The model under review builds one solid part; all positions refer to its coordinate system, in mm. Face numbers are marked on the shaded views. A direction names the side the tool comes from. Round coordinates to 2 decimals unless told otherwise and drop trailing zeros. Write each loop counter-clockwise with the first axis right and the second up, starting at its lowest first coordinate (ties: lowest second). Pieces come first, ordered by that corner, then holes. Notation, with made-up numbers: (-19, -22) -> (-8, -22) arc R19 ccw to (-8, -1) -> close; hole circle Ø5 at (60.5, -38.5). An arc over 180 degrees is marked (long way). Return JSON: item names as keys, results as strings. Group by question number.
1. For line 1 along X through (y, z) = (2.25, -6.5); line 2 along X through (y, z) = (-6.5, 0); line 3 along Y through (x, z) = (-7, 4.5), list the stretches that pass through material, from the lowest coordinate up. Write a range as from..to.
2. Clearance check with flat-ended pins moving along their axes: P1, Ø1, axis at y = -4, z = 7, coming from the -X side; P2, Ø1.5, axis at x = 10, y = 3, coming from the +Z side; P3, Ø4, axis at x = 1.5, y = -2.5, coming from the -Z side; P4, Ø4.5, axis at x = 0, z = 0, coming from the +Y side. State where each tip first meets the part, or that it passes through.
3. Mouldability with a two-part tool opening along Z and no side actions: class the marked faces 1, 2 and 3 as pulls with the +Z half, pulls with the -Z half, needs draft (parallel to the pull), parting line crosses it, or undercut.
4. Take a section at A-A, the plane y = -2.25. Write out the cut boundary in (x, z).
5. Take a section at B-B, the plane z = -11.5. Write out the cut boundary in (x, y).
6. Tool access review of the marked faces 4, 5 and 6: name each direction out of +Z, -Z, +X, -X, +Y, -Y from which nothing blocks a thin tool from reaching the whole face with its end or side.
from build123d import *

# Parameters (mm, degrees)
SKETCH1_R                 = 17
BOSS_EXTRUDE1_DEPTH       = 14
SKETCH9_W                 = 6
SKETCH9_H                 = 13.19
CUT_EXTRUDE1_DEPTH        = 28.820855486
SKETCH10_R                = 2.5
CUT_EXTRUDE2_DEPTH        = 6.35
FILLET2_R                 = 1
CIRPATTERN2_COUNT         = 3
FILLET2_OF_CIRPATTERN2_R  = 1
SKETCH12_R                = 20
CUT_EXTRUDE3_DEPTH        = 10
BOSS_EXTRUDE2_START       = 1
SKETCH13_R                = 17
BOSS_EXTRUDE2_DEPTH       = 1
M2X0_4_TAPPED_HOLE3_D     = 1.6
M2X0_4_TAPPED_HOLE3_DEPTH = 7
M2X0_4_TAPPED_HOLE3_TIP   = 0.480688495
FILLET3_R                 = 1
SKETCH14_R                = 11
SKETCH14_R_2              = 9.652
BOSS_EXTRUDE3_DEPTH       = 7
SKETCH20_R                = 2.5
CUT_EXTRUDE5_DEPTH        = 8
FILLET4_R                 = 0.25


with BuildPart() as part:
    # Sketch1 → Boss-Extrude1 (new body)
    with BuildSketch(Plane(origin=(0, 0, 0), x_dir=(1, 0, 0), z_dir=(0, 1, 0))):
        with Locations(Location((0, 0, 0), (0, 0, 270))):
            Circle(SKETCH1_R)
    extrude(amount=BOSS_EXTRUDE1_DEPTH)

    # Sketch9 → Cut-Extrude1 (cut, through all)
    with BuildSketch(Plane(origin=(0, 14, 0), x_dir=(1, 0, 0), z_dir=(0, 1, 0))):
        with Locations((0, 10.405)):
            Rectangle(SKETCH9_W, SKETCH9_H)
    cut_extrude1 = extrude(amount=-CUT_EXTRUDE1_DEPTH, mode=Mode.SUBTRACT)

    # Sketch10 → Cut-Extrude2 (cut, symmetric)
    with BuildSketch(Plane(origin=(0, 0, 0), x_dir=(0, 0, -1), z_dir=(1, 0, 0))):
        with Locations((11.5, 7)):
            Circle(SKETCH10_R)
    cut_extrude2 = extrude(amount=CUT_EXTRUDE2_DEPTH, both=True, mode=Mode.SUBTRACT)

    # Fillet2
    fillet2_edges = [part.edges().sort_by_distance(p)[0] for p in [
        (-3, 7, -3.81),
        (3, 7, -3.81),
    ]]
    fillet(fillet2_edges, radius=FILLET2_R)

    # CirPattern2: Cut-Extrude1, Cut-Extrude2 ×3 about axis
    cirpattern2_axis = Axis((0, 0, 0), (0, 1, 0))
    add([cut_extrude1.rotate(cirpattern2_axis, i * 360 / CIRPATTERN2_COUNT) for i in range(1, CIRPATTERN2_COUNT)], mode=Mode.SUBTRACT)
    add([cut_extrude2.rotate(cirpattern2_axis, i * 360 / CIRPATTERN2_COUNT) for i in range(1, CIRPATTERN2_COUNT)], mode=Mode.SUBTRACT)

    # Fillet2 of CirPattern2
    fillet2_of_cirpattern2_edges = [part.edges().sort_by_distance(p)[0] for p in [
        (-1.799556788, 7, 4.503076211),
        (-4.799556788, 7, -0.693076211),
        (4.799556788, 7, -0.693076211),
        (1.799556788, 7, 4.503076211),
    ]]
    fillet(fillet2_of_cirpattern2_edges, radius=FILLET2_OF_CIRPATTERN2_R)

    # Sketch12 → Cut-Extrude3 (cut)
    with BuildSketch(Plane(origin=(0, 7, 0), x_dir=(1, 0, 0), z_dir=(0, 1, 0))):
        Circle(SKETCH12_R)
    extrude(amount=CUT_EXTRUDE3_DEPTH, mode=Mode.SUBTRACT)

    # Sketch13 → Boss-Extrude2 (add)
    with BuildSketch(Plane.XZ.offset(BOSS_EXTRUDE2_START)):
        with Locations(Location((0, 0, 0), (0, 0, 270))):
            Circle(SKETCH13_R)
    extrude(amount=-BOSS_EXTRUDE2_DEPTH)

    # M2x0.4 Tapped Hole3
    with Locations(Plane(origin=(0, 7, 0), x_dir=(1, 0, 0), z_dir=(0, 1, 0))):
        with Locations((-11.258330249, 6.5), (11.258330249, 6.5), (0, -13), (-7.361215932, 4.25), (7.361215932, 4.25), (0, -8.5)):
            Hole(M2X0_4_TAPPED_HOLE3_D / 2, depth=M2X0_4_TAPPED_HOLE3_DEPTH)
            with Locations((0, 0, -(M2X0_4_TAPPED_HOLE3_DEPTH + M2X0_4_TAPPED_HOLE3_TIP / 2))):  # 118° drill point
                Cone(0, M2X0_4_TAPPED_HOLE3_D / 2, M2X0_4_TAPPED_HOLE3_TIP, mode=Mode.SUBTRACT)

    # Fillet3
    fillet3_edges = [part.edges().sort_by_distance(p)[0] for p in [
        (-10.828479469, 0, 2.787723921),
        (-4.906763147, 0, -0.292976634),
        (-3.299556788, 0, 1.905),
        (-2.199656366, 0, 4.395869853),
        (7.828479469, 0, 7.983876344),
        (2.199656366, 0, 4.395869853),
        (10.828479469, 0, 2.787723921),
        (4.906763147, 0, -0.292976634),
        (-3, 0, -10.771600265),
        (-2.707106781, 0, -4.102893219),
        (0, 0, -3.81),
        (2.707106781, 0, -4.102893219),
        (-7.828479469, 0, 7.983876344),
        (3.299556788, 0, 1.905),
        (3, 0, -10.771600265),
    ]]
    fillet(fillet3_edges, radius=FILLET3_R)

    # Sketch14 → Boss-Extrude3 (add)
    with BuildSketch(Plane.XZ.offset(1)):
        with Locations(Location((0, 0, 0), (0, 0, 270))):
            Circle(SKETCH14_R)
        with Locations(Location((0, 0, 0), (0, 0, 270))):
            Circle(SKETCH14_R_2, mode=Mode.SUBTRACT)
    extrude(amount=BOSS_EXTRUDE3_DEPTH)

    # Sketch20 → Cut-Extrude5 (cut)
    with BuildSketch(Plane.XZ.offset(1)):
        with Locations(Location((0, 0, 0), (0, 0, 270))):
            Circle(SKETCH20_R)
    extrude(amount=-CUT_EXTRUDE5_DEPTH, mode=Mode.SUBTRACT)

    # Fillet4
    fillet4_edges = [part.edges().sort_by_distance(p)[0] for p in [
        (-6.784292144, 4.5, 11.249261314),
        (-13.134292144, 4.5, 0.250738686),
        (13.134292144, 4.5, 0.250738686),
        (6.784292144, 4.5, 11.249261314),
        (-6.35, 4.5, -11.5),
        (6.35, 4.5, -11.5),
    ]]
    fillet(fillet4_edges, radius=FILLET4_R)


solid = part.part
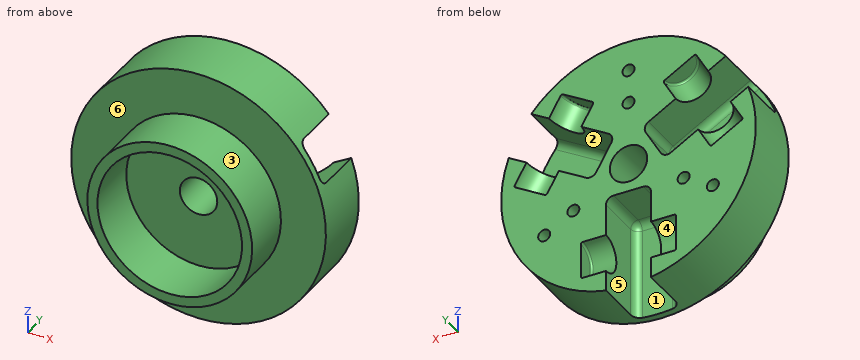
Output:
{
 "1": {"line 1": "x = -15.71..-12.06, -10.46..-3, 3..10.46, 12.06..15.71", "line 2": "x = -11..-9.65, 9.65..11", "line 3": "y = -1..0"},
 "2": {"P1": "stops at x = -8.87", "P2": "stops at z = 14.26", "P3": "stops at z = -17", "P4": "passes through"},
 "3": {"face 1": "needs draft", "face 2": "undercut", "face 3": "parting line crosses it"},
 "4": {"outline": "circle Ø22 at (0, 0); hole circle Ø19.3 at (0, 0)"},
 "5": {"outline": "(-12.52, -1) -> (12.52, -1) -> (12.52, 7) -> (6.35, 7) -> (6.35, 4.75) arc R0.25 cw to (6.1, 4.5) -> (3, 4.5) -> (3, 1) arc R1 cw to (2, 0) -> (-2, 0) arc R1 cw to (-3, 1) -> (-3, 4.5) -> (-6.1, 4.5) arc R0.25 cw to (-6.35, 4.75) -> (-6.35, 7) -> (-12.52, 7) -> close"},
 "6": {"face 4": "+Y", "face 5": "-Z, +Y", "face 6": "-Y"}
}
